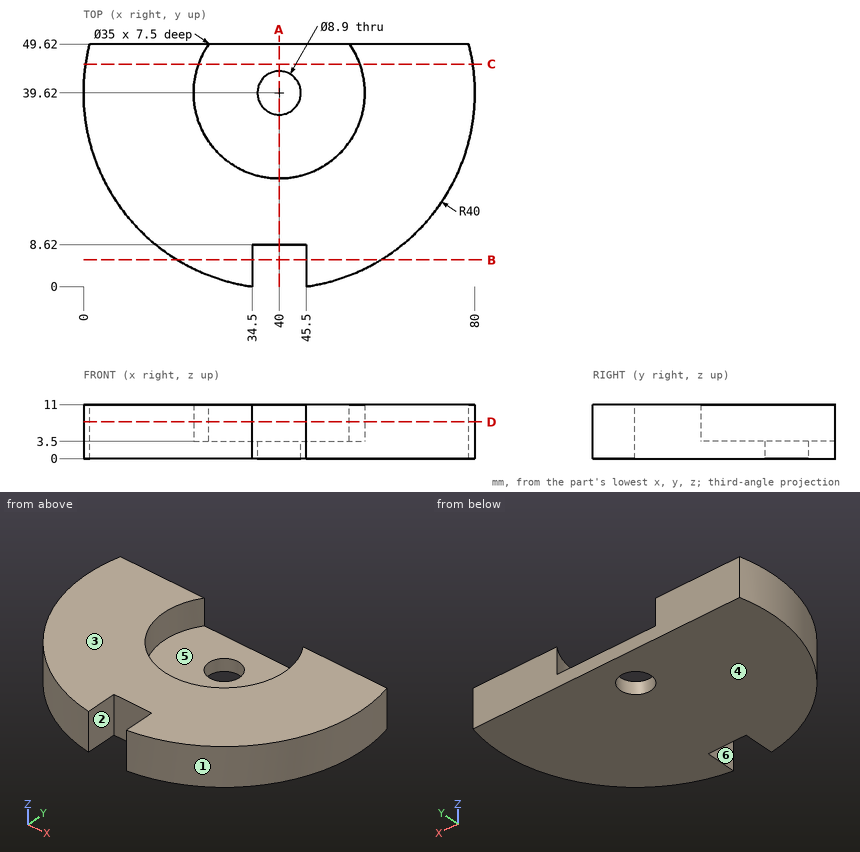
The drawing under review shows one solid part. Ordinate dimensions are in mm from its lowest x, y, z. A direction names the side the tool comes from. Coordinates: 2 decimals unless noted, no trailing zeros. Write each loop counter-clockwise with the first axis right and the second up, starting at its lowest first coordinate (ties: lowest second). Pieces come first, ordered by that corner, then holes. Notation, with made-up numbers: (27.5, 23) - (71.5, 23) arc R26 ccw to (71.5, 44) - close; hole circle Ø5 at (59, 17). An arc over 180 degrees is marked (long way). Answer as CSV lines item,"result".
(1) We need section A-A (x = 40). Give the boundary of the cut face in (y, z), plus the area to 3 significant figures.
Data:
outline,"(8.62, 0) - (35.17, 0) - (35.17, 3.5) - (22.12, 3.5) - (22.12, 11) - (8.62, 11) - close; (44.07, 0) - (49.62, 0) - (49.62, 3.5) - (44.07, 3.5) - close"
area,"214 mm2"
(2) We need section C-C (y = 45.5). Give the boundary of the cut face in (x, z).
Data:
outline,"(0.43, 0) - (79.57, 0) - (79.57, 11) - (56.48, 11) - (56.48, 3.5) - (23.52, 3.5) - (23.52, 11) - (0.43, 11) - close"
(3) Mouldability with a two-part tool opening along X and no side actions: class the marked faces 1, 2 and 3 as pulls with the +X half, pulls with the -X half, needs draft (parallel to the pull), parting line crosses it, or undercut.
Data:
face 1,"pulls with the +X half"
face 2,"undercut"
face 3,"needs draft"
(4) We need section D-D (z = 7.5). Give the boundary of the cut face in (x, y).
Data:
outline,"(1.27, 49.62) arc R40 ccw to (34.5, 0) - (34.5, 8.62) - (45.5, 8.62) - (45.5, 0) arc R40 ccw to (78.73, 49.62) - (54.36, 49.62) arc R17.5 cw (long way) to (25.64, 49.62) - close"
(5) For line 1 along X through (y, z) = (27.5, 4); line 2 along X through (y, z) = (23.5, 5.5); line 3 along Z through (x, y) = (42, 28), list the stretches that pass through material, from the lowest coordinate up. Write a range as [from, to].
Data:
line 1,"x = [1.88, 27.38], [52.62, 78.12]"
line 2,"x = [3.39, 33.19], [46.81, 76.61]"
line 3,"z = [0, 3.5]"
(6) Clearance check with flat-ended pins moving along their axes: pin 1 Ø4 at (x, z) = (16, 9.5) entering from -Y; pin 2 Ø6 at (x, z) = (69, 5) entering from -Y; pin 3 Ø5.5 at (x, z) = (42, 4) entering from -Y. State where each tip first meets the part, or that it passes through.
Data:
pin 1,"stops at y = 6.21"
pin 2,"stops at y = 9.22"
pin 3,"stops at y = 8.62"
(7) We need section B-B (y = 5.5). Give the boundary of the cut face in (x, z).
Data:
outline,"(19.12, 0) - (34.5, 0) - (34.5, 11) - (19.12, 11) - close; (45.5, 0) - (60.88, 0) - (60.88, 11) - (45.5, 11) - close"
(8) Tool access review of the marked faces 4, 5 and 6: name each direction out of +Z, -Z, +X, -X, +Y, -Y from which nothing blocks a thin tool from reaching the whole face with its end or side.
Data:
face 4,"-Z, +X, -X, +Y, -Y"
face 5,"+Z"
face 6,"+Z, -Z, -Y"
